CAD build for the part. Positions are in the model's coordinates, mm. Face numbers are marked on the shaded views. A direction names the side the tool comes from. Coordinates: 2 decimals unless noted, no trailing zeros. Order: outer loops, then holes, each group sorted by start corner. A loop starts at its lowest first (then second) coordinate and runs counter-clockwise, first axis right, second up. Notation, with made-up numbers: M 29,-1 L 85,-1 A9 ccw 85,12 Z; hole C 16,-12.5 d3. An arc over 180 degrees is marked long. Write item = value, one per line.
from build123d import *

# Parameters (mm, degrees)
SKETCH002_R     = 8.1
PAD001_DEPTH    = 5
SKETCH_W        = 15
SKETCH_H        = 30
PAD_DEPTH       = 12.1
SKETCH001_R     = 6.2
POCKET_DEPTH    = 15.001
SKETCH003_R     = 1.5
POCKET001_DEPTH = 12.101
SKETCH004_R     = 2.8
POCKET002_DEPTH = 3
SKETCH005_W     = 30
SKETCH005_H     = 12.1
PAD002_DEPTH    = 2.5
SKETCH006_R     = 8.2
POCKET003_DEPTH = 2.5


with BuildPart() as pad001:
    # Sketch002 → Pad001 (new body, symmetric)
    with BuildSketch(Plane.YZ):
        with Locations((0, 12)):
            Circle(SKETCH002_R)
    extrude(amount=PAD001_DEPTH, both=True)


with BuildPart() as pocket003:
    # Sketch → Pad (new body)
    with BuildSketch(Plane.XY):
        Rectangle(SKETCH_W, SKETCH_H)
    extrude(amount=PAD_DEPTH)

    # Sketch001 → Pocket (cut, through all)
    with BuildSketch(Plane.YZ.offset(7.5)):
        with Locations((0, 12)):
            Circle(SKETCH001_R)
    extrude(amount=-POCKET_DEPTH, mode=Mode.SUBTRACT)

    # Cut: cut Pad001
    add(pad001.part, mode=Mode.SUBTRACT)

    # Sketch003 → Pocket001 (cut, through all)
    with BuildSketch(Plane(origin=(0, 0, 0), x_dir=(1, 0, 0), z_dir=(0, 0, -1))):
        with Locations((0.026833, -11.5)):
            Circle(SKETCH003_R)
        with Locations((0, 11.5)):
            Circle(SKETCH003_R)
    extrude(amount=-POCKET001_DEPTH, mode=Mode.SUBTRACT)

    # Sketch004 → Pocket002 (cut)
    with BuildSketch(Plane(origin=(0, 0, 0), x_dir=(1, 0, 0), z_dir=(0, 0, -1))):
        with Locations((0, 11.5)):
            Circle(SKETCH004_R)
        with Locations((0, -11.5)):
            Circle(SKETCH004_R)
    extrude(amount=-POCKET002_DEPTH, mode=Mode.SUBTRACT)

    # Sketch005 → Pad002 (new body)
    with BuildSketch(Plane.YZ.offset(7.5)):
        with Locations((0, 6.05)):
            Rectangle(SKETCH005_W, SKETCH005_H)
    extrude(amount=PAD002_DEPTH)

    # Sketch006 → Pocket003 (cut)
    with BuildSketch(Plane.YZ.offset(10)):
        with Locations((0, 12.1)):
            Circle(SKETCH006_R)
    extrude(amount=-POCKET003_DEPTH, mode=Mode.SUBTRACT)


solid = pocket003.part
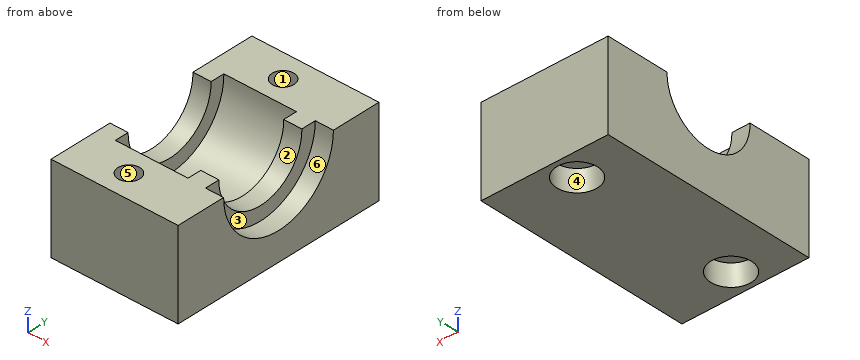
(1) Slice it at D-D, the plane y = 0. Write the cut outline in (x, z), then the cut area to 4 significant figures.
Evaluation:
outline = M -7.5,0 L 10,0 L 10,3.9 L 7.5,3.9 L 7.5,5.8 L 5,5.8 L 5,3.9 L -5,3.9 L -5,5.8 L -7.5,5.8 Z
area = 77.75 mm²
(2) Pull direction X, two halves, no side cores. Call the marked faces 1, 2 and 3: +X half, -X half, draft (parallel to the pull), parting line (faces both ways), or undercut.
Evaluation:
face_1 = undercut
face_2 = draft
face_3 = +X half
(3) Slice it at B-B, the plane z = 9.5. Write the cut outline in (x, y).
Evaluation:
outline = M -7.5,-15 L 10,-15 L 10,-7.78 L 7.5,-7.78 L 7.5,-5.67 L 5,-5.67 L 5,-7.7 L -5,-7.7 L -5,-5.67 L -7.5,-5.67 Z; M -7.5,5.67 L -5,5.67 L -5,7.7 L 5,7.7 L 5,5.67 L 7.5,5.67 L 7.5,7.78 L 10,7.78 L 10,15 L -7.5,15 Z; hole C 0,-11.5 d3; hole C 0.03,11.5 d3
(4) Slice it at A-A, the plane y = -11.5. Write the cut outline in (x, z).
Evaluation:
outline = M -7.5,0 L -2.8,0 L -2.8,3 L -1.5,3 L -1.5,12.1 L -7.5,12.1 Z; M 1.5,3 L 2.8,3 L 2.8,0 L 10,0 L 10,12.1 L 1.5,12.1 Z
(5) Pin check, flat tips, straight feed: pin 1 Ø6.5 at (y, z) = (3.5, 9) entering from +X; pin 2 Ø3 at (x, y) = (-0.5, -10.5) entering from -Z. Stop position of each tip, or through.
Evaluation:
pin_1 = 7.5
pin_2 = 3
(6) Wall check: line 1 (Y direction, x = 0, z = 1.7); line 2 (X direction, y = -11.5, z = 9.25); line 3 (X direction, y = 5.5, z = 8.5). Give the ranges that are in metal, low to high. Write a range as from..to.
Evaluation:
line_1 = -15..-14.3, -8.7..8.7, 14.3..15
line_2 = -7.5..-1.5, 1.5..10
line_3 = -7.5..-5, 5..7.5
(7) Tool access for the marked faces 4, 5 and 6: list every direction of +Z, -Z, +X, -X, +Y, -Y with a clear straight run to the whole face (end or side of a thin tool).
Evaluation:
face_4 = -Z
face_5 = +Z, -Z
face_6 = +Z, +X
(8) Slice it at C-C, the plane x = 1. Write the cut outline in (y, z).
Evaluation:
outline = M -15,0 L -14.12,0 L -14.12,3 L -12.62,3 L -12.62,12.1 L -15,12.1 Z; M -10.38,3 L -8.88,3 L -8.88,0 L 8.88,0 L 8.88,3 L 10.36,3 L 10.36,12.1 L 8.1,12.1 A8.1 cw long -8.1,12.1 L -10.38,12.1 Z; M 12.64,3 L 14.12,3 L 14.12,0 L 15,0 L 15,12.1 L 12.64,12.1 Z
